Drawing for the job (mm, zero at the part's lowest x, y, z). A direction names the side the tool comes from. Round coordinates to 2 decimals unless told otherwise and drop trailing zeros. Write each loop counter-clockwise with the first axis right and the second up, starting at its lowest first coordinate (ties: lowest second). Pieces come first, ordered by that corner, then holes.
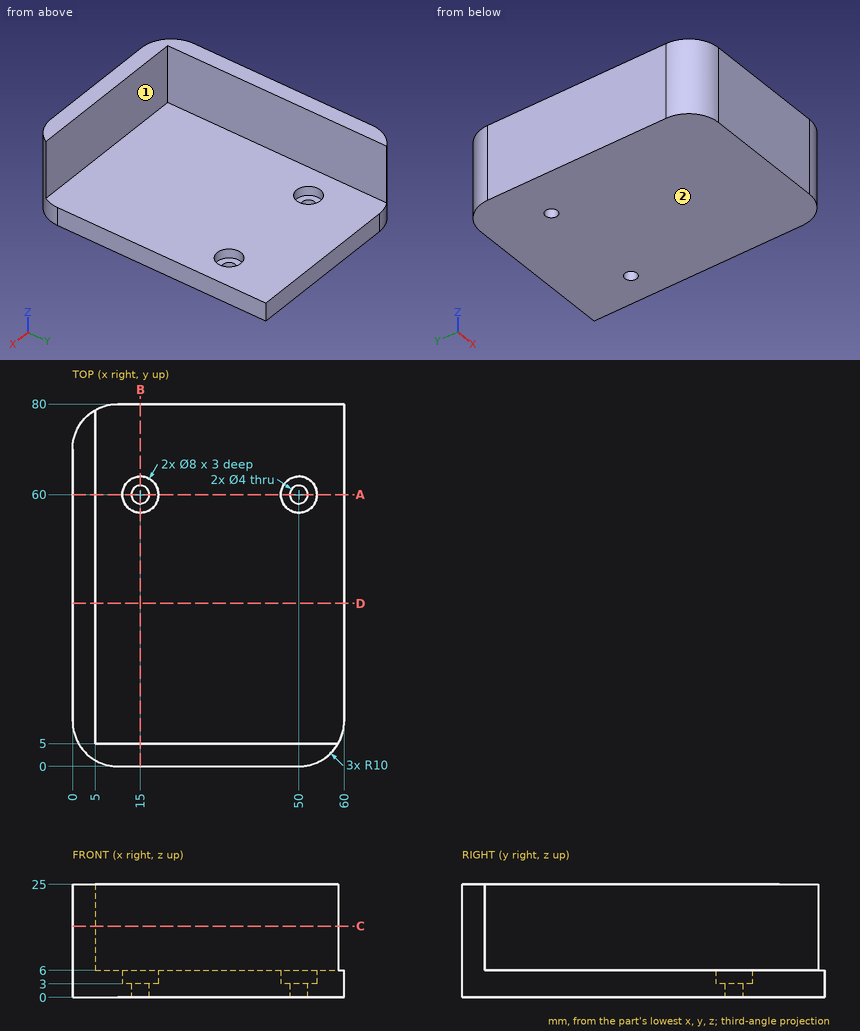
Q1. Drop flat-ended pins along their axis: P1, Ø4, axis at x = 50, y = 61.5, coming from the +Z side; P2, Ø6, axis at y = 44, z = 10.5, coming from the +X side; P3, Ø5, axis at x = 13, z = 14.5, coming from the +Y side. Give the stop position or say it passes through.
Q2. Saw through at D-D, the plane y = 36. Write the cut outline in (x, z).
Q3. Saw through at C-C, the plane z = 15.75. Write the cut outline in (x, y).
Q4. Wall check: line 1 (X direction, y = 60, z = 5.2); line 2 (Y direction, x = 50, z = 4); line 3 (Y direction, x = 50, z = 1.5). Give the ranges that are in metal, low to high.
Q5. Saw through at A-A, the plane y = 60. Write the cut outline in (x, z), and give its area (3 significant figures).
Q6. Tool access for the marked faces 1 and 2: list every direction of +Z, -Z, +X, -X, +Y, -Y with a clear straight run to the whole face (end or side of a thin tool).
Q7. Saw through at B-B, the plane x = 15. Write the cut outline in (y, z).
Computed:
1. P1: stops at z = 3
1. P2: stops at x = 5
1. P3: stops at y = 5
2. outline: (0, 0) - (60, 0) - (60, 6) - (5, 6) - (5, 25) - (0, 25) - close
3. outline: (0, 10) arc R10 ccw to (10, 0) - (50, 0) arc R10 ccw to (58.66, 5) - (5, 5) - (5, 78.66) arc R10 ccw to (0, 70) - close
4. line 1: x = 0 to 11, 19 to 46, 54 to 60
4. line 2: y = 0 to 56, 64 to 80
4. line 3: y = 0 to 58, 62 to 80
5. outline: (0, 0) - (13, 0) - (13, 3) - (11, 3) - (11, 6) - (5, 6) - (5, 25) - (0, 25) - close; (17, 0) - (48, 0) - (48, 3) - (46, 3) - (46, 6) - (19, 6) - (19, 3) - (17, 3) - close; (52, 0) - (60, 0) - (60, 6) - (54, 6) - (54, 3) - (52, 3) - close
5. area: 383 mm2
6. face 1: +Z, +X, +Y
6. face 2: -Z, +X, -X, +Y, -Y
7. outline: (0, 0) - (58, 0) - (58, 3) - (56, 3) - (56, 6) - (5, 6) - (5, 25) - (0, 25) - close; (62, 0) - (80, 0) - (80, 6) - (64, 6) - (64, 3) - (62, 3) - close
